from build123d import *

# Parameters (mm, degrees)
BOSS_EXTRUDE1_DEPTH = 3.9


with BuildPart() as part:
    # Sketch1 → Boss-Extrude1 (new body)
    with BuildSketch(Plane(origin=(0, 0, 0), x_dir=(1, 0, 0), z_dir=(0, 1, 0))):
        with BuildLine():
            Line((-4.02, 3.65), (4.02, 3.65))
            ThreePointArc((4.02, 3.65), (7.67, 0), (4.02, -3.65))
            Line((4.02, -3.65), (-4.02, -3.65))
            ThreePointArc((-4.02, -3.65), (-7.67, 0), (-4.02, 3.65))
        make_face()
        Polygon((3.12, 2.4), (3.12, 0.9), (1.62, 0.9), (1.62, -0.9), (3.12, -0.9), (3.12, -2.4), (4.92, -2.4), (4.92, -0.9), (6.42, -0.9), (6.42, 0.9), (4.92, 0.9), (4.92, 2.4), align=None, mode=Mode.SUBTRACT)
        Polygon((-4.870347538, 2.400403287), (-4.870347538, 0.900403287), (-6.370347538, 0.900403287), (-6.370347538, -0.899596713), (-4.870347538, -0.899596713), (-4.870347538, -2.399596713), (-3.070347538, -2.399596713), (-3.070347538, -0.899596713), (-1.570347538, -0.899596713), (-1.570347538, 0.900403287), (-3.070347538, 0.900403287), (-3.070347538, 2.400403287), align=None, mode=Mode.SUBTRACT)
    extrude(amount=BOSS_EXTRUDE1_DEPTH)


solid = part.part
Geometry check sheet. Reference: the model listing, model coordinates, mm. A direction names the side the tool comes from. Round coordinates to 2 decimals unless told otherwise and drop trailing zeros. Loops run counter-clockwise (first coordinate to the right, second up) from the corner with the lowest first, then second, coordinate; pieces in that order, holes last. Notation, with made-up numbers: (-9.5, 84) - (12.5, 84) arc R33 ccw to (12.5, 118) - close; hole circle Ø2 at (73.5, 54). An arc over 180 degrees is marked (long way). One line per question, with ' | ' between items. Start each with the question number.
1. Cross-section at C-C on y = 0.3. Record the cut outline in (x, z).
2. Draft check along X on faces 1 (the face through (-7.67, 1.92, 0.08)), 2 (the face through (-3.07, 2, -2)), 3 (the face through (0, 3.9, 0)). Enter one of: released by +X, released by -X, zero draft, split by the parting line, or undercut.
3. Cross-section at A-A on z = 0. Record the cut outline in (x, y), then the cut area to 3 significant figures.
4. Tool access check on faces 4 (the face through (0, 2, 3.65)), 5 (the face through (4.92, 2, 2)). Record the directions out of +Z, -Z, +X, -X, +Y, -Y that give a thin tool (end or side, any length) a straight path to the whole face; none if there is none.
5. Depth check by flat-ended pin: pin 1 (0.8 mm diameter, centred on y = 3, z = 1.5, fed in from -X); pin 2 (1.2 mm diameter, centred on x = 5.5, y = 1.5, fed in from +Z); pin 3 (1.2 mm diameter, centred on y = 1.5, z = 2, fed in from +X). Enter the tip coordinate at first touch or a pass-through.
6. Cross-section at B-B on x = 2.5. Record the cut outline in (y, z), then the cut area to 4 significant figures.
7. Cross-section at D-D on z = 1.75. Record the cut outline in (x, y), then the cut area to 3 significant figures.
8. Scan lines: line 1 (Z direction, x = -3, y = 0.9); line 2 (X direction, y = 1.2, z = -2.25); line 3 (X direction, y = 1.8, z = -0.25). Record each from-to range of solid material in increasing order. Write a range as [from, to].
Taken from the geometry:
1) outline: (-4.02, -3.65) - (4.02, -3.65) arc R3.65 ccw to (4.02, 3.65) - (-4.02, 3.65) arc R3.65 ccw to start; hole (-6.37, -0.9) - (-4.87, -0.9) - (-4.87, -2.4) - (-3.07, -2.4) - (-3.07, -0.9) - (-1.57, -0.9) - (-1.57, 0.9) - (-3.07, 0.9) - (-3.07, 2.4) - (-4.87, 2.4) - (-4.87, 0.9) - (-6.37, 0.9) - close; hole (1.62, -0.9) - (3.12, -0.9) - (3.12, -2.4) - (4.92, -2.4) - (4.92, -0.9) - (6.42, -0.9) - (6.42, 0.9) - (4.92, 0.9) - (4.92, 2.4) - (3.12, 2.4) - (3.12, 0.9) - (1.62, 0.9) - close
2) face 1: released by -X | face 2: undercut | face 3: zero draft
3) outline: (-7.67, 0) - (-6.37, 0) - (-6.37, 3.9) - (-7.67, 3.9) - close; (-1.57, 0) - (1.62, 0) - (1.62, 3.9) - (-1.57, 3.9) - close; (6.42, 0) - (7.67, 0) - (7.67, 3.9) - (6.42, 3.9) - close | area: 22.4 mm²
4) face 4: +Z, +X, -X, +Y, -Y | face 5: +Y, -Y
5) pin 1: x = -7.5 | pin 2: z = 3.54 | pin 3: x = 7.39
6) outline: (0, -3.65) - (3.9, -3.65) - (3.9, -0.9) - (0, -0.9) - close; (0, 0.9) - (3.9, 0.9) - (3.9, 3.65) - (0, 3.65) - close | area: 21.45 mm²
7) outline: (-7.22, 0) - (-4.87, 0) - (-4.87, 3.9) - (-7.22, 3.9) - close; (-3.07, 0) - (3.12, 0) - (3.12, 3.9) - (-3.07, 3.9) - close; (4.92, 0) - (7.22, 0) - (7.22, 3.9) - (4.92, 3.9) - close | area: 42.3 mm²
8) line 1: [-3.65, -0.9], [0.9, 3.65] | line 2: [-6.89, -4.87], [-3.07, 3.12], [4.92, 6.89] | line 3: [-7.66, -6.37], [-1.57, 1.62], [6.42, 7.66]
